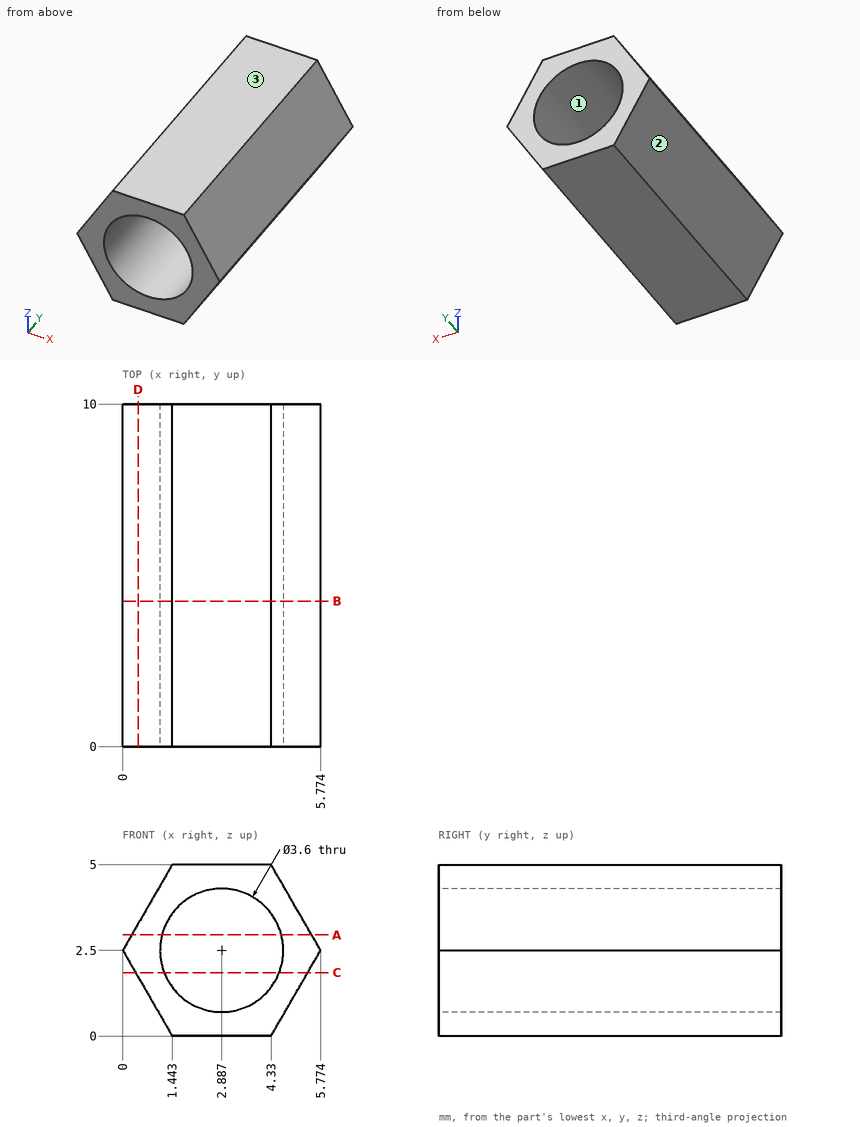
The figure shows three views and two pictorial views of one solid part (mm, origin at its lowest corner). Answer the questions. Round coordinates to 2 decimals unless told otherwise and drop trailing zeros. Loops run counter-clockwise (first coordinate to the right, second up) from the corner with the lowest first, then second, coordinate; pieces in that order, holes last. Notation, with made-up numbers: (65.25, 17) - (101.25, 17) arc R35 ccw to (101.25, 49) - close; hole circle Ø8 at (79, -3.5). An arc over 180 degrees is marked (long way). Use one line per item in the form item = value. Start each with the question number.
(1) Find section B-B on y = 4.25. Determine the outline of the cut face in (x, z).
(2) Find section C-C on z = 1.85. Determine the outline of the cut face in (x, y) (1 decimal).
(3) Flat-ended cylindrical pins translate along their axes: P1, Ø3, axis at x = 3, z = 1, coming from the +Y side; P2, Ø1.5, axis at y = 8.5, z = 2, coming from the -X side. Find the tip coordinate at first contact, or state that the pin passes through.
(4) Find section D-D on x = 0.45. Determine the outline of the cut face in (y, z), and give its area (3 significant figures).
(5) Find section A-A on z = 2.95. Determine the outline of the cut face in (x, y).
(6) Determine the mould class of the marked faces 1, 2 and 3 for opening direction X: +X half, -X half, draft (parallel to the pull), parting line (faces both ways), or undercut.
(7) Consider line 1 (Z direction, x = 3.3, y = 6); line 2 (X direction, y = 1.75, z = 3.3) (1 decimal); line 3 (X direction, y = 7.5, z = 3.9) (1 decimal). Determine where each line is inside the solid, lowest interval first.
Answer list:
q1.outline = (0, 2.5) - (1.44, 0) - (4.33, 0) - (5.77, 2.5) - (4.33, 5) - (1.44, 5) - close; hole circle Ø3.6 at (2.89, 2.5)
q2.outline = (0.4, 0) - (1.2, 0) - (1.2, 10) - (0.4, 10) - close; (4.6, 0) - (5.4, 0) - (5.4, 10) - (4.6, 10) - close
q3.P1 = 10
q3.P2 = 0
q4.outline = (0, 1.72) - (10, 1.72) - (10, 3.28) - (0, 3.28) - close
q4.area = 15.6 mm^2
q5.outline = (0.26, 0) - (1.14, 0) - (1.14, 10) - (0.26, 10) - close; (4.63, 0) - (5.51, 0) - (5.51, 10) - (4.63, 10) - close
q6.face_1 = undercut
q6.face_2 = -X half
q6.face_3 = draft
q7.line_1 = 0 to 0.75, 4.25 to 5
q7.line_2 = 0.5 to 1.3, 4.5 to 5.3
q7.line_3 = 0.8 to 1.8, 4 to 5
